The model under review builds one solid part; all positions refer to its coordinate system, in mm. A direction names the side the tool comes from. Give positions to 0.01 mm unless a question says otherwise; leave off trailing zeros. Loops run counter-clockwise (first coordinate to the right, second up) from the corner with the lowest first, then second, coordinate; pieces in that order, holes last. Notation, with made-up numbers: M -5.75,15 L 13.25,15 A17 cw 13.25,38 Z; hole C 7,12 d2. An arc over 180 degrees is marked long. Write item = value, one per line. Start each with the question number.
1. Wall thickness on line 1 along Z through (x, y) = (4, 0.4); line 2 along Y through (x, z) = (4, -0.2); line 3 along Y through (x, z) = (0.9, 4): over which ranges is each line inside the solid? List them lowest first. Write a range as from..to.
2. Draft analysis for pull direction Y (two halves, no side actions). For faces 4 (the face through (6, 2.7, -0.8)), 5 (the face through (1, 5, 4)), 6 (the face through (5.5, 7.5, -0.5)), 7 (the face through (3.263, 5.676, -0.493)), state which applies: pulls with the +Y half, pulls with the -Y half, needs draft (parallel to the pull), parting line crosses it, or undercut.
3. For pin 1 (1.6 mm diameter, centred on x = 1, z = 2.5, fed in from -Y); pin 2 (1.2 mm diameter, centred on x = 4, y = 5, fed in from +Z); pin 3 (1.5 mm diameter, centred on x = 0.5, y = 1.5, fed in from -Z); pin 4 (4.5 mm diameter, centred on y = 6.5, z = 3, fed in from +X), all flat-tipped, find the tip position at first contact; note any pin that passes through.
4. We need section D-D on y = 7.5. Give the boundary of the cut face in (x, z), then the cut area to 3 significant figures.
5. For faces 1 (the face through (2, 5.6, 1.8)), 2 (the face through (2, 0.5, -2)), 3 (the face through (5, 1, -2)), list the 3-axis set-ups (+Z, -Z, +X, -X, +Y, -Y) from which the entire face can be reached by the end or side of a thin tool; tool diameter is ignored.
6. We need section A-A on x = 3.6. Give the boundary of the cut face in (y, z).
7. We need section B-B on z = -2.5. Give the boundary of the cut face in (x, y).
8. We need section C-C on y = 5.5. Give the boundary of the cut face in (x, z).
from build123d import *

# Parameters (mm, degrees)
SKETCH1_R           = 1
BOSS_EXTRUDE1_DEPTH = 1
SKETCH2_R           = 1
BOSS_EXTRUDE2_DEPTH = 1
BOSS_EXTRUDE3_DEPTH = 2
CUT_EXTRUDE1_DEPTH  = 2


with BuildPart() as part:
    # Sketch1 → Boss-Extrude1 (new body)
    with BuildSketch(Plane.XY):
        Polygon((5, 8), (6, 7), (6, 0), (0, 0), (0, 8), align=None)
        with Locations((4, 5)):
            Circle(SKETCH1_R, mode=Mode.SUBTRACT)
    extrude(amount=-BOSS_EXTRUDE1_DEPTH)

    # Sketch2 → Boss-Extrude2 (add)
    with BuildSketch(Plane.XZ):
        with BuildLine():
            Line((6, -1), (6, -2.999291988))
            ThreePointArc((6, -2.999291988), (4, -4.999291988), (2, -2.999291988))
            Line((2, -2.999291988), (2, -1))
            Line((2, -1), (6, -1))
        make_face()
        with Locations((4, -2.999291988)):
            Circle(SKETCH2_R, mode=Mode.SUBTRACT)
    extrude(amount=-BOSS_EXTRUDE2_DEPTH)

    # Sketch3 → Boss-Extrude3 (add)
    with BuildSketch(Plane.ZY):
        with BuildLine():
            Line((0, 8), (0, 4))
            Line((0, 4), (4.678841552, 4))
            Line((4.678841552, 4), (4.678841552, 5))
            Line((4.678841552, 5), (2.884219665, 5))
            ThreePointArc((2.884219665, 5), (1.884219665, 6), (2.884219665, 7))
            Line((2.884219665, 7), (4.678841552, 7))
            Line((4.678841552, 7), (4.678841552, 8))
            Line((4.678841552, 8), (0, 8))
        make_face()
    extrude(amount=-BOSS_EXTRUDE3_DEPTH)

    # Sketch4 → Cut-Extrude1 (cut)
    with BuildSketch(Plane(origin=(0, 8, 0), x_dir=(1, 0, 0), z_dir=(0, 1, 0))):
        Polygon((1, -4.678841552), (2, -2.678841552), (2, -4.678841552), align=None)
    extrude(amount=-CUT_EXTRUDE1_DEPTH, mode=Mode.SUBTRACT)


solid = part.part
Final values:
q1.line_1 = -5..-4, -2..0
q1.line_2 = 0..4, 6..8
q1.line_3 = 4..5, 7..8
q2.face_4 = needs draft
q2.face_5 = undercut
q2.face_6 = pulls with the +Y half
q2.face_7 = undercut
q3.pin_1 = 4
q3.pin_2 = through
q3.pin_3 = -1
q3.pin_4 = 2
q4.outline = M 0,-1 L 5.5,-1 L 5.5,0 L 2,0 L 2,2.68 L 1,4.68 L 0,4.68 Z
q4.area = 13.9 mm²
q5.face_1 = +Z, +X, +Y, -Y
q5.face_2 = -Z, -X, +Y, -Y
q5.face_3 = -Z, +X, -X, +Y
q6.outline = M 0,-4.96 L 1,-4.96 L 1,-3.92 L 0,-3.92 Z; M 0,-2.08 L 1,-2.08 L 1,-1 L 4.08,-1 L 4.08,0 L 0,0 Z; M 5.92,-1 L 8,-1 L 8,0 L 5.92,0 Z
q7.outline = M 2,0 L 3.13,0 L 3.13,1 L 2,1 Z; M 4.87,0 L 6,0 L 6,1 L 4.87,1 Z
q8.outline = M 0,-1 L 3.13,-1 L 3.13,0 L 2,0 L 2,2.02 L 0,2.02 Z; M 4.87,-1 L 6,-1 L 6,0 L 4.87,0 Z
